Here's the drawing with two shaded views (mm, measured from the low corner). I have some questions. A direction names the side the tool comes from. Round coordinates to 2 decimals unless told otherwise and drop trailing zeros. Loops run counter-clockwise (first coordinate to the right, second up) from the corner with the lowest first, then second, coordinate; pieces in that order, holes last. Notation, with made-up numbers: M 35,-38 L 56,-38 A30 cw 56,-5 Z; hole C 14.5,82 d11. An arc over 180 degrees is marked long. One line per item, written item: value. Start each with the question number.
Q1. I'm going to push flat-ended pins straight in: pin 1 Ø2 at (x, y) = (6, 2) entering from -Z; pin 2 Ø0.9 at (y, z) = (3, 3.5) entering from -X; pin 3 Ø3 at (y, z) = (1, 1.5) entering from -X. Where does each tip first touch, or does it pass through?
Q2. Imagine slicing it at C-C (z = 4.3). Please give me the cut outline in (x, y), then the cut area to 3 significant figures.
Q3. Please list where these lines run through material, in increasing order: line 1 along X through (y, z) = (3.95, 2.95); line 2 along X through (y, z) = (4.3, 3.25); line 3 along Z through (x, y) = (0.5, 4.65).
Q4. Thinking about a two-plate mould opening in Z: for the marked faces 1, 2, 3 and 4, which applies, released by +Z, released by -Z, zero draft, split by the parting line, or undercut?
Q5. Imagine slicing it at A-A (y = 3). Please give me the cut outline in (x, z), then the cut area to 3 significant figures.
Q6. Imagine slicing it at D-D (x = 5.25). Please give me the cut outline in (y, z).
Q7. Imagine slicing it at B-B (x = 0.5). Please give me the cut outline in (y, z), then the cut area to 3 significant figures.
Q8. Which directions (+Z, -Z, +X, -X, +Y, -Y) give clear straight access to the entire face, cutting with the end or side of a thin tool? Please do the marked faces 5 and 6.
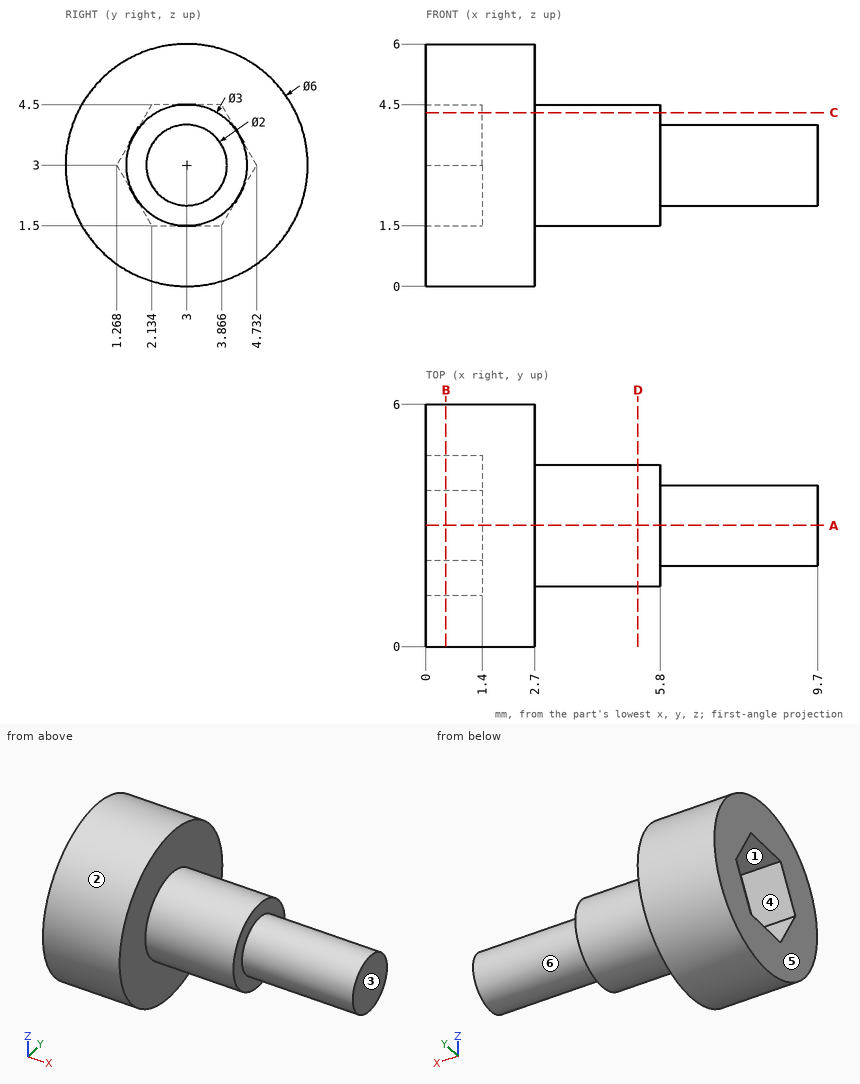
Report:
1. pin 1: stops at z = 1.5
1. pin 2: stops at x = 1.4
1. pin 3: stops at x = 0
2. outline: M 0,0.3 L 2.7,0.3 L 2.7,2.25 L 5.8,2.25 L 5.8,3.75 L 2.7,3.75 L 2.7,5.7 L 0,5.7 L 0,3.98 L 1.4,3.98 L 1.4,2.02 L 0,2.02 Z
2. area: 16.5 mm²
3. line 1: x = 1.4 to 9.7
3. line 2: x = 1.4 to 5.8
3. line 3: z = 0.49 to 2.86, 3.14 to 5.51
4. face 1: undercut
4. face 2: split by the parting line
4. face 3: zero draft
4. face 4: undercut
5. outline: M 0,0 L 2.7,0 L 2.7,1.5 L 5.8,1.5 L 5.8,2 L 9.7,2 L 9.7,4 L 5.8,4 L 5.8,4.5 L 2.7,4.5 L 2.7,6 L 0,6 L 0,4.5 L 1.4,4.5 L 1.4,1.5 L 0,1.5 Z
5. area: 29.1 mm²
6. outline: C 3,3 d3
7. outline: C 3,3 d6; hole M 1.27,3 L 2.13,1.5 L 3.87,1.5 L 4.73,3 L 3.87,4.5 L 2.13,4.5 Z
7. area: 20.5 mm²
8. face 5: +Z, -Z, -X, +Y, -Y
8. face 6: +X
